Can you work these out from the model? Positions are in its coordinate system, mm. A direction names the side the tool comes from. Give positions to 0.01 mm unless a question says otherwise; leave off trailing zeros. Order: outer loops, then holes, each group sorted by start corner. A loop starts at its lowest first (then second) coordinate and runs counter-clockwise, first axis right, second up. Notation, with made-up numbers: (51, 71.5) - (72, 71.5) arc R20 cw to (72, 95.5) - close; hole circle Ø4 at (23.5, -37.75). An arc over 180 degrees is marked (long way). Return JSON: item names as keys, results as strings.
```python
from build123d import *

# Parameters (mm, degrees)
F0_W           = 41
F0_H           = 41
F1_DEPTH       = 12
F2_D           = 3.3
F2_DEPTH       = 20
F2_CBORE_D     = 6.5
F2_CBORE_DEPTH = 3
F2_TIP         = 0.9914200214
F3_W           = 39
F3_H           = 39
F4_DEPTH       = 8
F5_R           = 5
F6_W           = 10
F6_H           = 8
F7_DEPTH       = 1
F8_R           = 1


with BuildPart() as f1:
    # F0 (on Top) → F1 (new body)
    with BuildSketch(Plane.XY):
        with Locations((-7.3711453006, 4.3136782655)):
            Rectangle(F0_W, F0_H)
    extrude(amount=F1_DEPTH)

    # F2
    with Locations(Plane(origin=(0, 0, 0), x_dir=(1, 0, 0), z_dir=(0, 0, -1))):
        with Locations((8.1288546994, -19.8136782655), (-22.8711453006, -19.8136782655), (-22.8711453006, 11.1863217345), (8.1288546994, 11.1863217345)):
            CounterBoreHole(F2_D / 2, F2_CBORE_D / 2, F2_CBORE_DEPTH, depth=F2_DEPTH)
            with Locations((0, 0, -(F2_DEPTH + F2_TIP / 2))):  # 118° drill point
                Cone(0, F2_D / 2, F2_TIP, mode=Mode.SUBTRACT)

    # F3 (on face) → F4 (cut)
    with BuildSketch(Plane.XY.offset(12)):
        with Locations((-7.3711453006, 4.3136782655)):
            Rectangle(F3_W, F3_H)
    extrude(amount=-F4_DEPTH, mode=Mode.SUBTRACT)

    # F5
    f5_edges = [f1.edges().sort_by_distance(p)[0] for p in [
        (13.128855, -16.186322, 6),
        (12.128855, -15.186322, 8),
        (-27.871145, -16.186322, 6),
        (-26.871145, -15.186322, 8),
        (-27.871145, 24.813678, 6),
        (-26.871145, 23.813678, 8),
        (13.128855, 24.813678, 6),
        (12.128855, 23.813678, 8),
    ]]
    fillet(f5_edges, radius=F5_R)

    # F6 (on face) → F7 (cut, through all)
    with BuildSketch(Plane.YZ.offset(13.1288546994)):
        with Locations((4.3136782655, 8)):
            Rectangle(F6_W, F6_H)
    extrude(amount=-F7_DEPTH, mode=Mode.SUBTRACT)

    # F8
    f8_edges = [f1.edges().sort_by_distance(p)[0] for p in [
        (12.628855, 9.313678, 4),
        (12.628855, -0.686322, 4),
    ]]
    fillet(f8_edges, radius=F8_R)


solid = f1.part
```
1. If I drill on L1, parallel to Y at x = -14, z = 11.25; L2, parallel to X at y = -3, z = 6.75; L3, parallel to X at y = 22, z = 2.25, over which ranges is the centre line in solid material (lowest first)? Write a range as [from, to].
Checks:
{"L1": "[-16.19, -15.19], [23.81, 24.81]", "L2": "[-27.87, -26.87], [12.13, 13.13]", "L3": "[-27.37, -25.28], [-20.47, 5.72], [10.53, 12.63]"}
2. Suppose I cut it at A-A (z = 2.5). List the corners of the cut face in (x, y) for me, plus the area to 3 significant figures.
Checks:
{"outline": "(-27.87, -11.19) arc R5 ccw to (-22.87, -16.19) - (8.13, -16.19) arc R5 ccw to (13.13, -11.19) - (13.13, 19.81) arc R5 ccw to (8.13, 24.81) - (-22.87, 24.81) arc R5 ccw to (-27.87, 19.81) - close; hole circle Ø6.5 at (-22.87, -11.19); hole circle Ø6.5 at (-22.87, 19.81); hole circle Ø6.5 at (8.13, -11.19); hole circle Ø6.5 at (8.13, 19.81)", "area": "1,530 mm^2"}
3. Thinking about a two-plate mould opening in Y: for faces 1 (the face through (12.129, 15, 8)), 2 (the face through (-27.871, 4, 6)), 3 (the face through (11.625, -14.761, 6.084)), 4 (the face through (-25.368, 22.388, 7.944)), which applies, +Y half, -Y half, draft (parallel to the pull), parting line (faces both ways), or undercut?
Checks:
{"face 1": "undercut", "face 2": "draft", "face 3": "-Y half", "face 4": "undercut"}
4. Suppose I cut it at D-D (z = 7.25). List the corners of the cut face in (x, y) for me, plus the area to 3 significant figures.
Checks:
{"outline": "(-27.87, -11.19) arc R5 ccw to (-22.87, -16.19) - (8.13, -16.19) arc R5 ccw to (13.13, -11.19) - (13.13, -0.69) - (12.13, -0.69) - (12.13, -10.19) arc R5 cw to (7.13, -15.19) - (-21.87, -15.19) arc R5 cw to (-26.87, -10.19) - (-26.87, 18.81) arc R5 cw to (-21.87, 23.81) - (7.13, 23.81) arc R5 cw to (12.13, 18.81) - (12.13, 9.31) - (13.13, 9.31) - (13.13, 19.81) arc R5 ccw to (8.13, 24.81) - (-22.87, 24.81) arc R5 ccw to (-27.87, 19.81) - close", "area": "150 mm^2"}
5. On a 3-axis mill with a long thin cutter (end or side, diameter ignored), from which of +Z, -Z, +X, -X, +Y, -Y can I reach the whole of each face in a straight line? I mean faces 5 (the face through (12.6, 9.314, 8.5)), 6 (the face through (-8, -15.186, 8)), 7 (the face through (-19.77, -12.16, 1.48)). Say none if no direction works.
Checks:
{"face 5": "+Z, +X", "face 6": "+Z", "face 7": "-Z"}
6. Suppose I cut it at C-C (x = -4.5). List the corners of the cut face in (y, z) for me, plus the area to 3 significant figures.
Checks:
{"outline": "(-16.19, 0) - (24.81, 0) - (24.81, 12) - (23.81, 12) - (23.81, 4) - (-15.19, 4) - (-15.19, 12) - (-16.19, 12) - close", "area": "180 mm^2"}
7. For pin 1 Ø1.5 at (x, y) = (-2.5, 17.5) entering from -Z; pin 2 Ø0.5 at (x, z) = (12.5, 10) entering from +Y; pin 3 Ø1.5 at (y, z) = (8, 6) entering from +X; pin 4 Ø1.5 at (x, y) = (7.5, 0) entering from +Z, each with a flat end and sliding along its axis, tell me the tip position at first contact or that it passes through.
Checks:
{"pin 1": "z = 0", "pin 2": "y = 22.64", "pin 3": "x = -26.87", "pin 4": "z = 4"}
8. Suppose I cut it at B-B (y = 6). List the corners of the cut face in (x, z) for me, plus the area to 3 significant figures.
Checks:
{"outline": "(-27.87, 0) - (13.13, 0) - (13.13, 4) - (-26.87, 4) - (-26.87, 12) - (-27.87, 12) - close", "area": "172 mm^2"}
